```python
from build123d import *

# Parameters (mm, degrees)
F0_R     = 9.6
F1_DEPTH = 15.8
F2_R     = 5.4
F3_DEPTH = 20
F4_R     = 14.45
F5_DEPTH = 3.7
F6_R     = 5.4
F7_DEPTH = 3.7


with BuildPart() as f1:
    # F0 (on Top) → F1 (new body)
    with BuildSketch(Plane.XY):
        Circle(F0_R)
    extrude(amount=F1_DEPTH)

    # F2 (on Top) → F3 (cut)
    with BuildSketch(Plane.XY):
        Circle(F2_R)
    extrude(amount=F3_DEPTH, mode=Mode.SUBTRACT)

    # F4 (on Top) → F5 (join)
    with BuildSketch(Plane.XY):
        Circle(F4_R)
    extrude(amount=F5_DEPTH)

    # F6 (on Top) → F7 (cut)
    with BuildSketch(Plane.XY):
        Circle(F6_R)
    extrude(amount=F7_DEPTH, mode=Mode.SUBTRACT)


solid = f1.part
```
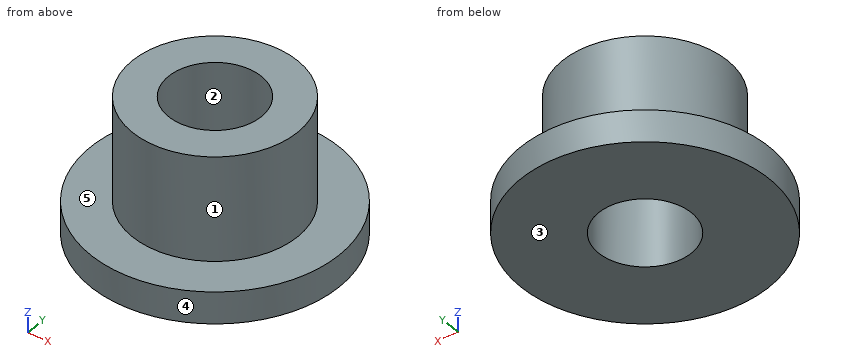
Input: part model. Units: mm. Frame: model coordinates. Face numbers are marked on the shaded views. A direction names the side the tool comes from. Coordinates: 2 decimals unless noted, no trailing zeros. Write each loop counter-clockwise with the first axis right and the second up, starting at its lowest first coordinate (ties: lowest second). Pieces come first, ordered by that corner, then holes. Notation, with made-up numbers: (24, 59) -> (59, 59) arc R25 ccw to (59, 81) -> close; hole circle Ø5 at (62, 23.25). An arc over 180 degrees is marked (long way). Write each question's results on one line, items separated by ' | '.
Item 1: Section query C-C on z = 2.25. Return loops of the section in (x, y), plus the area to 3 significant figures.
Conclusion:
outline: circle Ø28.9 at (0, 0); hole circle Ø10.8 at (0, 0) | area: 564 mm^2
Item 2: Pin query (flat end, axial travel): pin 1 Ø1 at (x, y) = (-10.5, -8) entering from +Z; pin 2 Ø4 at (y, z) = (7, 2) entering from +X; pin 3 Ø6 at (y, z) = (9, 8) entering from +X. Return the tip coordinate at first contact, or that it passes through.
Conclusion:
pin 1: stops at z = 3.7 | pin 2: stops at x = 13.56 | pin 3: stops at x = 7.49
Item 3: Section query D-D on x = -9. Return loops of the section in (y, z), plus the area to 3 significant figures.
Conclusion:
outline: (-11.3, 0) -> (11.3, 0) -> (11.3, 3.7) -> (3.34, 3.7) -> (3.34, 15.8) -> (-3.34, 15.8) -> (-3.34, 3.7) -> (-11.3, 3.7) -> close | area: 165 mm^2
Item 4: Section query B-B on x = -3.75. Return loops of the section in (y, z).
Conclusion:
outline: (-13.95, 0) -> (-3.89, 0) -> (-3.89, 15.8) -> (-8.84, 15.8) -> (-8.84, 3.7) -> (-13.95, 3.7) -> close; (3.89, 0) -> (13.95, 0) -> (13.95, 3.7) -> (8.84, 3.7) -> (8.84, 15.8) -> (3.89, 15.8) -> close
Item 5: Section query A-A on y = 0. Return loops of the section in (x, z), plus the area to 3 significant figures.
Conclusion:
outline: (-14.45, 0) -> (-5.4, 0) -> (-5.4, 15.8) -> (-9.6, 15.8) -> (-9.6, 3.7) -> (-14.45, 3.7) -> close; (5.4, 0) -> (14.45, 0) -> (14.45, 3.7) -> (9.6, 3.7) -> (9.6, 15.8) -> (5.4, 15.8) -> close | area: 169 mm^2
Item 6: Material intervals for probe 1 along Y at (x, z) = (0, 5); probe 2 along Y at (x, z) = (-3.75, 10), sorted ascending.
Conclusion:
probe 1: y = -9.6 to -5.4, 5.4 to 9.6 | probe 2: y = -8.84 to -3.89, 3.89 to 8.84
Item 7: Set-up query: the marked faces 4 and 5. Return all of +Z, -Z, +X, -X, +Y, -Y with unobstructed straight access to the full face (end or side cutting, diameter ignored); none if empty.
Conclusion:
face 4: +Z, -Z | face 5: +Z
Item 8: Mould query, pull axis Y, two halves, no side actions, for the marked faces 1, 2 and 3. Classes: +Y half, -Y half, draft (parallel to the pull), parting line (faces both ways), or undercut.
Conclusion:
face 1: parting line | face 2: undercut | face 3: draft
